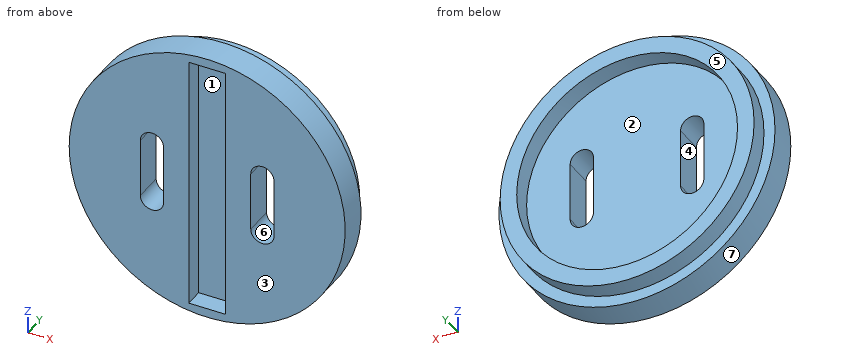
Autodesk Inventor part; units mm, degrees
ref_plane "YZ Plane" through (0, 0, 0) normal (1, 0, 0) x (0, 1, 0)
ref_plane "XZ Plane" through (0, 0, 0) normal (0, 1, 0) x (-1, 0, 0)
ref_plane "XY Plane" through (0, 0, 0) normal (0, 0, 1) x (1, 0, 0)
sketch "Sketch1" plane through (0, 0, 0) normal (0, 1, 0) x (-1, 0, 0)
  circle A0 centre (0, 0) radius 34.5
  circle A1 centre (0, 0) radius 37.5
  circle A2 centre (0, 0) radius 30
  line L0 (15, 8) -> (15, -8) construction
  line L1 (11.8377, 8) -> (11.8377, -8)
  line L2 (18.1623, -8) -> (18.1623, 8)
  arc A3 (18.1623, 8) -> (11.8377, 8) centre (15, 8) ccw
  arc A4 (11.8377, -8) -> (18.1623, -8) centre (15, -8) ccw
  line L3 (0, 16.7478) -> (0, 6) construction
  line L4 (-11.8377, 8) -> (-11.8377, -8)
  line L5 (-18.1623, -8) -> (-18.1623, 8)
  arc A5 (-11.8377, 8) -> (-18.1623, 8) centre (-15, 8) ccw
  arc A6 (-18.1623, -8) -> (-11.8377, -8) centre (-15, -8) ccw
  point P0 (15, 0)
  dimension "d0" = 69
  dimension "d1" = 75
  dimension "d2" = 60
  dimension "d3" = 15
  dimension "d4" = 16
  dimension "d5" = 8
  dimension "d6" = 3.1623
  dimension "d7" = 6
  dimension "d8" = 15
  dimension "d9" = 16.7478
extrude "Extrusion1" add sketch "Sketch1" against normal blind 8 contours A0 | A1 | A2
extrude "Extrusion2" add sketch "Sketch1" along normal blind 5 contours A0
sketch "Sketch2" plane through (0, -8, 0) normal (0, -1, 0) x (1, 0, 0)
  line L0 (-5, 35) -> (5, 35)
  line L1 (5, 35) -> (5, -35)
  line L2 (5, -35) -> (-5, -35)
  line L3 (-5, -35) -> (-5, 35)
  line L4 (-5, 35) -> (5, -35) construction
  line L5 (5, 35) -> (-5, -35) construction
  point P0 (0, 0)
  point P1 (0, 35)
  dimension "d16" = 10
  dimension "d17" = 70
extrude "Extrusion3" cut sketch "Sketch2" against normal blind 5
properties part number "bay_bottom"
Check sheet for the modelled part. Datum: model origin and axes. Units: mm. Face numbers are marked on the shaded views. A direction names the side the tool comes from. Round coordinates to 2 decimals unless told otherwise and drop trailing zeros. Order: outer loops, then holes, each group sorted by start corner. A loop starts at its lowest first (then second) coordinate and runs counter-clockwise, first axis right, second up.
Q1. Draft check along X on the marked faces 5, 6 and 7. Enter one of: pulls with the +X half, pulls with the -X half, needs draft (parallel to the pull), parting line crosses it, or undercut.
Filled sheet:
face 5: needs draft
face 6: undercut
face 7: parting line crosses it
Q2. Scan lines: L1, parallel to X at y = -3.25, z = -3; L2, parallel to X at y = -4.5, z = 3.5; L3, parallel to Z at x = 0, y = 2.5. Record each from-to range of solid material in increasing order.
Filled sheet:
L1: x = -37.38 to -18.16, -11.84 to -5, 5 to 11.84, 18.16 to 37.38
L2: x = -37.34 to -18.16, -11.84 to -5, 5 to 11.84, 18.16 to 37.34
L3: z = -34.5 to -30, 30 to 34.5
Q3. Set-up check for the marked faces 1, 2, 3 and 4: record each of +Z, -Z, +X, -X, +Y, -Y from which the full face is reachable in a straight line by a thin tool's end or side.
Filled sheet:
face 1: -Y
face 2: +Y
face 3: +Z, -Z, +X, -X, -Y
face 4: +Y, -Y
Q4. Cross-section at B-B, the plane x = 0. Enter the section's corners in (y, z).
Filled sheet:
outline: (-8, -37.5) - (0, -37.5) - (0, -34.5) - (5, -34.5) - (5, -30) - (0, -30) - (0, 30) - (5, 30) - (5, 34.5) - (0, 34.5) - (0, 37.5) - (-8, 37.5) - (-8, 35) - (-3, 35) - (-3, -35) - (-8, -35) - close
Q5. Cross-section at C-C, the plane y = -1.75. Enter the section's corners in (x, z).
Filled sheet:
outline: circle Ø75 at (0, 0); hole (-18.16, -8) arc R3.16 ccw to (-11.84, -8) - (-11.84, 8) arc R3.16 ccw to (-18.16, 8) - close; hole (11.84, -8) arc R3.16 ccw to (18.16, -8) - (18.16, 8) arc R3.16 ccw to (11.84, 8) - close
Q6. Cross-section at D-D, the plane x = 15. Enter the section's corners in (y, z).
Filled sheet:
outline: (-8, -34.37) - (0, -34.37) - (0, -31.07) - (5, -31.07) - (5, -25.98) - (0, -25.98) - (0, -11.16) - (-8, -11.16) - close; (-8, 11.16) - (0, 11.16) - (0, 25.98) - (5, 25.98) - (5, 31.07) - (0, 31.07) - (0, 34.37) - (-8, 34.37) - close
Q7. Cross-section at A-A, the plane z = 0. Enter the section's corners in (x, y).
Filled sheet:
outline: (-37.5, -8) - (-18.16, -8) - (-18.16, 0) - (-30, 0) - (-30, 5) - (-34.5, 5) - (-34.5, 0) - (-37.5, 0) - close; (-11.84, -8) - (-5, -8) - (-5, -3) - (5, -3) - (5, -8) - (11.84, -8) - (11.84, 0) - (-11.84, 0) - close; (18.16, -8) - (37.5, -8) - (37.5, 0) - (34.5, 0) - (34.5, 5) - (30, 5) - (30, 0) - (18.16, 0) - close
Q8. Depth check by flat-ended pin: P1, Ø5, axis at y = 1.5, z = 5, coming from the -X side; P2, Ø1.5, axis at y = -5.5, z = -17, coming from the -X side; P3, Ø22.5, axis at x = -18, z = -4, coming from the +Y side. Enter the tip coordinate at first touch or a pass-through.
Filled sheet:
P1: stops at x = -37.38
P2: stops at x = -33.8
P3: stops at y = 0
